```python
from build123d import *

# Parameters (mm, degrees)
F1_DEPTH = 228
F3_DEPTH = 30
F4_R     = 1
F6_R     = 0.5
F7_R     = 0.5


# Not quite as in the source:
# - two fillets or chamfers of one size are made in one step
# - a pattern or mirror of a feature is missing from the dataset's text; its kind, count and spacing are read off the source's solid


with BuildPart() as f1:
    # F0 (on Top) → F1 (new body, symmetric)
    with BuildSketch(Plane.XY):
        Polygon((-14, 0.5), (-17, 0.5), (-20, -2.5), (20, -2.5), (17, 0.5), (14, 0.5), (11, 0.5), (-11, 0.5), align=None)
        Polygon((-14, 25.5), (-14, 0.5), (-11, 0.5), (-11, 4), (-11, 7), (-11, 25.5), align=None)
        Polygon((11, 4), (11, 0.5), (14, 0.5), (14, 25.5), (11, 25.5), (11, 7), align=None)
        Polygon((-11, 7), (-11, 4), (-5, 4), (-5, 7), (-5, 15), (-8, 15), (-8, 7), align=None)
        Polygon((5, 4), (11, 4), (11, 7), (8, 7), (8, 15), (5, 15), (5, 7), align=None)
    extrude(amount=F1_DEPTH, both=True)

    # F2 (on Right) → F3 (cut, symmetric)
    with BuildSketch(Plane.YZ):
        Polygon((25.5, 228), (0.5, 228), (-2.5, 228), (25.5, 200), align=None)
    f3 = extrude(amount=F3_DEPTH, both=True, mode=Mode.SUBTRACT)

    # F3_copies: F3 across plane
    add(f3.mirror(Plane(origin=(0, 0, 0), x_dir=(-1, 0, 0), z_dir=(0, 0, -1))), mode=Mode.SUBTRACT)

    # F4
    f4_edges = [f1.edges().sort_by_distance(p)[0] for p in [
        (17, 0.5, 0),
        (12.5, 25.5, 200),
        (-11, 0.5, 0),
        (-12.5, 25.5, 200),
        (-17, 0.5, 0),
        (11, 0.5, 0),
        (6.5, 15, 210.5),
        (-6.5, 15, 210.5),
        (12.5, 25.5, -200),
        (6.5, 15, -210.5),
        (-6.5, 15, -210.5),
        (-12.5, 25.5, -200),
        (5, 4, 0),
        (-5, 4, 0),
    ]]
    fillet(f4_edges, radius=F4_R)

    # F6
    f6_edges = [f1.edges().sort_by_distance(p)[0] for p in [
        (8, 7, 0),
        (-11, 7, 0),
        (-11, 4, 0),
        (11, 4, 0),
        (11, 7, 0),
        (-8, 7, 0),
    ]]
    fillet(f6_edges, radius=F6_R)

    # F7
    f7_edges = [f1.edges().sort_by_distance(p)[0] for p in [
        (-20, -2.5, 0),
        (20, -2.5, 0),
        (14, 0.5, 0),
        (-14, 0.5, 0),
    ]]
    fillet(f7_edges, radius=F7_R)


solid = f1.part
```
Source: CAD feature listing. Evaluate the final solid. Frame: model axes, mm. A direction names the side the tool comes from. Round coordinates to 2 decimals unless told otherwise and drop trailing zeros. Answer as a JSON object with one key per item and string values. Group by question number.
(1) Mould query, pull axis X, two halves, no side actions, for faces 1 (the flat face through (0, 0.5, 3)), 2 (the flat face through (14, 13, 3)), 3 (the flat face through (8, 11, 3)), 4 (the flat face through (0, -2.5, 3)). Classes: +X half, -X half, draft (parallel to the pull), parting line (faces both ways), or undercut.
(2) Ray query, line 1 (X direction, y = 7.75, z = -133); line 2 (Y direction, x = 7.5, z = -171); line 3 (X direction, y = 6.5, z = -118.5). Return the intervals inside material, ascending. Write a range as [from, to].
(3) First-contact query: pin 1 (3 mm diameter, centred on x = -5, z = -1, fed in from +Y); pin 2 (7.5 mm diameter, centred on y = 16, z = -79, fed in from -X); pin 3 (3 mm diameter, centred on y = 11.5, z = 31, fed in from +X). Flat tips, straight axial feed; report the tip coordinate or a pass-through.
(4) Reachability of faces 5 (the flat face through (5.8, 6.2, -219.3)), 6 (the flat face through (-14, 13, 3)), 7 (the flat face through (11, 17, 3)) from +Z, -Z, +X, -X, +Y, -Y: full face, straight path, thin tool, end or side. Return the list, or none.
Computed values:
{
 "1": {"face 1": "undercut", "face 2": "+X half", "face 3": "undercut", "face 4": "draft"},
 "2": {"line 1": "[-14, -11], [-8, -5], [5, 8], [11, 14]", "line 2": "[-2.5, 0.5], [4, 15]", "line 3": "[-14, -5], [5, 14]"},
 "3": {"pin 1": "y = 15", "pin 2": "x = -14", "pin 3": "x = 14"},
 "4": {"face 5": "-Z, +X, -X, +Y", "face 6": "+Z, -Z, -X, +Y", "face 7": "+Z, -Z, +Y"}
}
